The drawing under review shows one solid part. Ordinate dimensions are in mm from its lowest x, y, z. Give positions to 0.01 mm unless a question says otherwise; leave off trailing zeros. Loops run counter-clockwise (first coordinate to the right, second up) from the corner with the lowest first, then second, coordinate; pieces in that order, holes last. Notation, with made-up numbers: (70.25, -22) - (117.25, -22) arc R27 ccw to (117.25, 16) - close; hole circle Ø6 at (14.5, 41). An arc over 180 degrees is marked (long way). Put each result on its own line as item: value. Start each with the question number.
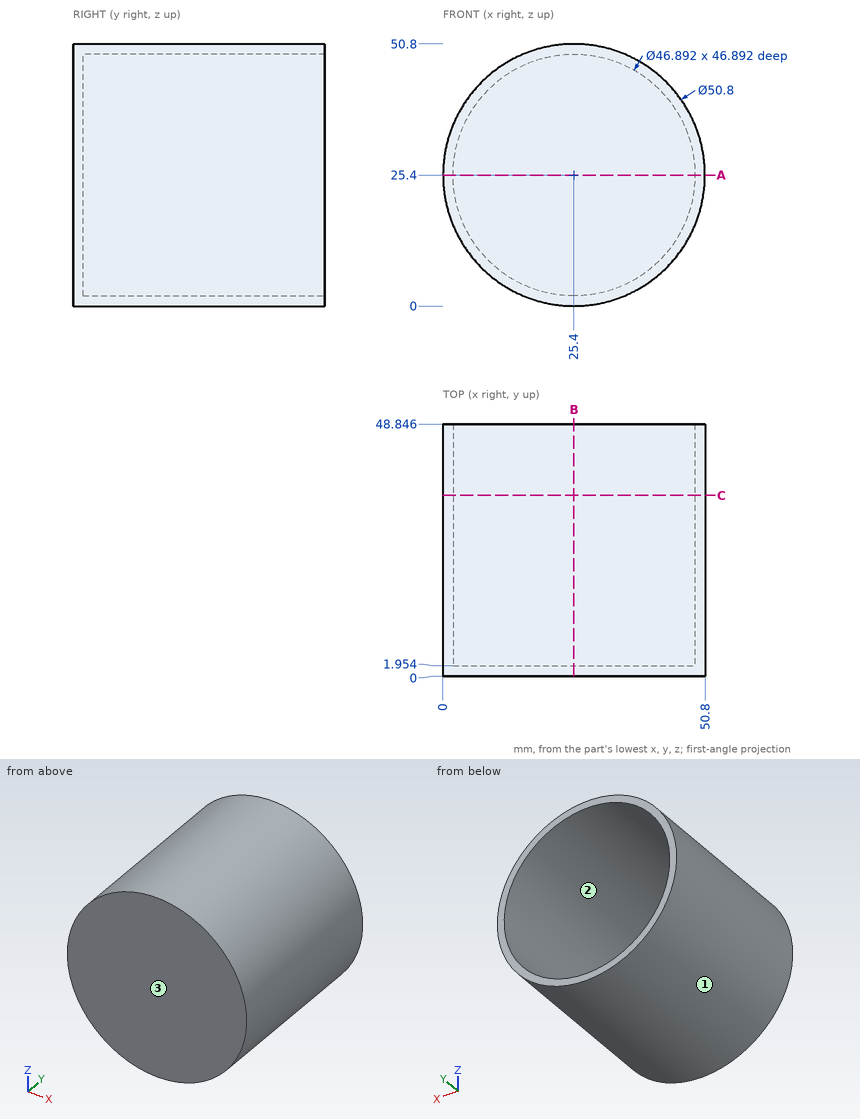
Item 1: Consider section B-B (x = 25.4). State the section outline as (y, z) points.
Item 2: Consider section A-A (z = 25.4). State the section outline as (x, y) points.
Item 3: For P1, Ø1, axis at x = 24.5, z = 17.5, coming from the +Y side; P2, Ø8, axis at x = 7, z = 35, coming from the +Y side; P3, Ø1.5, axis at y = 35.5, z = 19, coming from the -X side; P4, Ø10, axis at y = 8.5, z = 35, coming from the -X side, all flat-tipped, find the tip position at first contact; note any pin that passes through.
Item 4: Mouldability with a two-part tool opening along X and no side actions: class the marked faces 1, 2 and 3 as pulls with the +X half, pulls with the -X half, needs draft (parallel to the pull), parting line crosses it, or undercut.
Item 5: Consider section C-C (y = 35). State the section outline as (x, z) points.
Item 6: For L1, parallel to X at y = 29, z = 25; L2, parallel to Y at x = 4, z = 23.5, list the stretches that pass through material, from the lowest coordinate up. Write a range as from..to.
Geometry says:
1. outline: (0, 0) - (48.85, 0) - (48.85, 1.95) - (1.95, 1.95) - (1.95, 48.85) - (48.85, 48.85) - (48.85, 50.8) - (0, 50.8) - close
2. outline: (0, 0) - (50.8, 0) - (50.8, 48.85) - (48.85, 48.85) - (48.85, 1.95) - (1.95, 1.95) - (1.95, 48.85) - (0, 48.85) - close
3. P1: stops at y = 1.95
3. P2: stops at y = 48.85
3. P3: stops at x = 0.64
3. P4: stops at x = 0.42
4. face 1: parting line crosses it
4. face 2: undercut
4. face 3: needs draft
5. outline: circle Ø50.8 at (25.4, 25.4); hole circle Ø46.89 at (25.4, 25.4)
6. L1: x = 0..1.96, 48.84..50.8
6. L2: y = 0..1.95
